For this review, take the finished solid that the model builds, in its own axes (mm). A direction names the side the tool comes from. Round coordinates to 2 decimals unless told otherwise and drop trailing zeros. Order: outer loops, then holes, each group sorted by start corner. A loop starts at its lowest first (then second) coordinate and runs counter-clockwise, first axis right, second up. Notation, with made-up numbers: M 65,-29 L 119,-29 A10 cw 119,-14 Z; hole C -26.5,87.25 d1. An arc over 180 degrees is marked long. Write item = value, one per line. Start each with the question number.
from build123d import *

# Parameters (mm, degrees)
SKETCH_1_R      = 50.5
SKETCH_1_R_2    = 2.6
SKETCH_1_R_3    = 35
EXTRUDE_1_DEPTH = 2
SKETCH_3_R      = 2.55
SKETCH_3_R_2    = 12
EXTRUDE_4_DEPTH = 2
FILLET_2_R      = 3


with BuildPart() as part:
    # 草图1 → 凸台-拉伸1 (new body)
    with BuildSketch(Plane.XY):
        Circle(SKETCH_1_R)
        with Locations((0, 40)):
            Circle(SKETCH_1_R_2, mode=Mode.SUBTRACT)
        Circle(SKETCH_1_R_3, mode=Mode.SUBTRACT)
        with Locations((28.284271247, 28.284271247)):
            Circle(SKETCH_1_R_2, mode=Mode.SUBTRACT)
        with Locations((40, 0)):
            Circle(SKETCH_1_R_2, mode=Mode.SUBTRACT)
        with Locations((28.284271247, -28.284271247)):
            Circle(SKETCH_1_R_2, mode=Mode.SUBTRACT)
        with Locations((0, -40)):
            Circle(SKETCH_1_R_2, mode=Mode.SUBTRACT)
        with Locations((-28.284271247, -28.284271247)):
            Circle(SKETCH_1_R_2, mode=Mode.SUBTRACT)
        with Locations((-40, 0)):
            Circle(SKETCH_1_R_2, mode=Mode.SUBTRACT)
        with Locations((-28.284271247, 28.284271247)):
            Circle(SKETCH_1_R_2, mode=Mode.SUBTRACT)
    extrude(amount=EXTRUDE_1_DEPTH)

    # 草图3 → 凸台-拉伸4 (add)
    with BuildSketch(Plane(origin=(0, 0, 0), x_dir=(-1, 0, 0), z_dir=(0, 0, -1))):
        with BuildLine():
            Line((-5, 34.641016151), (-5, 21.424285286))
            ThreePointArc((-5, 21.424285286), (-19.052558883, 11), (-21.053975315, -6.382015624))
            Line((-21.053975315, -6.382015624), (-32.5, -12.990381057))
            ThreePointArc((-32.5, -12.990381057), (-30.310889132, -17.5), (-27.5, -21.650635095))
            Line((-27.5, -21.650635095), (-16.053975315, -15.042269662))
            ThreePointArc((-16.053975315, -15.042269662), (0, -22), (16.053975315, -15.042269662))
            Line((16.053975315, -15.042269662), (27.5, -21.650635095))
            ThreePointArc((27.5, -21.650635095), (30.310889132, -17.5), (32.5, -12.990381057))
            Line((32.5, -12.990381057), (21.053975315, -6.382015624))
            ThreePointArc((21.053975315, -6.382015624), (19.052558883, 11), (5, 21.424285286))
            Line((5, 21.424285286), (5, 34.641016151))
            ThreePointArc((5, 34.641016151), (0, 35), (-5, 34.641016151))
        make_face()
        with Locations((0, 17.5)):
            Circle(SKETCH_3_R, mode=Mode.SUBTRACT)
        with Locations((0, -17.5)):
            Circle(SKETCH_3_R, mode=Mode.SUBTRACT)
        with Locations((-15.155444566, -8.75)):
            Circle(SKETCH_3_R, mode=Mode.SUBTRACT)
        with Locations((15.155444566, -8.75)):
            Circle(SKETCH_3_R, mode=Mode.SUBTRACT)
        with Locations((-15.155444566, 8.75)):
            Circle(SKETCH_3_R, mode=Mode.SUBTRACT)
        Circle(SKETCH_3_R_2, mode=Mode.SUBTRACT)
        with Locations((15.155444566, 8.75)):
            Circle(SKETCH_3_R, mode=Mode.SUBTRACT)
    extrude(amount=-EXTRUDE_4_DEPTH)

    # 圆角2
    fillet_2_edges = [part.edges().sort_by_distance(p)[0] for p in [
        (5, 21.424285286, 1),
        (5, 34.641016151, 1),
        (-5, 34.641016151, 1),
        (-5, 21.424285286, 1),
        (-21.053975315, -6.382015624, 1),
        (-32.5, -12.990381057, 1),
        (-27.5, -21.650635095, 1),
        (-16.053975315, -15.042269662, 1),
        (16.053975315, -15.042269662, 1),
        (27.5, -21.650635095, 1),
        (32.5, -12.990381057, 1),
        (21.053975315, -6.382015624, 1),
    ]]
    fillet(fillet_2_edges, radius=FILLET_2_R)


solid = part.part
(1) For line 1 along Y through (x, z) = (-25, 0.5); line 2 along X through (y, z) = (15.5, 1.4); line 3 along Y through (x, z) = (27, 0.2), list the stretches that pass through material, from the lowest coordinate up.
(2) We need section B-B, the plane x = 0. Write out the cut boundary in (y, z), then the cut area to 3 significant figures.
(3) Insertion check: pin 1 (4.5 mm diameter, centred on x = 28.28, y = 28.28, fed in from -Z); pin 2 (1 mm diameter, centred on y = 27, z = 1.5, fed in from -X). Each pin has a flat end and moves straight along its axis. Give the tip position at first contact, or say it passes through.
(4) For faces 1 (the flat face through (11, -11, 2)), 2 (the flat face through (21.217, -18.023, 0.986)), list the 3-axis set-ups (+Z, -Z, +X, -X, +Y, -Y) from which the entire face can be reached by the end or side of a thin tool; tool diameter is ignored.
(5) We need section A-A, the plane y = 0. Write out the cut boundary in (x, z).
(6) We need section D-D, the plane y = 17.5. Write out the cut boundary in (x, z).
(7) Draft analysis for pull direction X (two halves, no side actions). For faces 3 (the flat face through (11, -11, 0)), 4 (the flat face through (-26.217, -9.363, 0.986)), 5 (the cylindrical face through (29.68, -26.09, 0.99)), 6 (the cylindrical face through (-10.95, -49.3, 0.99)), state which applies: released by +X, released by -X, zero draft, split by the parting line, or undercut.
(8) We need section C-C, the plane y = 40. Write out the cut boundary in (x, z), then the cut area to 3 significant figures.
Values:
q1.line_1 = -43.88 to -24.49, -20.35 to -8.66, 24.49 to 43.88
q1.line_2 = -48.06 to -31.38, -15.61 to -1.58, 1.58 to 15.61, 31.38 to 48.06
q1.line_3 = -42.68 to -30.54, -26.02 to -9.81, 22.27 to 26.02, 30.54 to 42.68
q2.outline = M -50.5,0 L -42.6,0 L -42.6,2 L -50.5,2 Z; M -37.4,0 L -35,0 L -35,2 L -37.4,2 Z; M -22,0 L -20.05,0 L -20.05,2 L -22,2 Z; M -14.95,0 L -12,0 L -12,2 L -14.95,2 Z; M 12,0 L 14.95,0 L 14.95,2 L 12,2 Z; M 20.05,0 L 37.4,0 L 37.4,2 L 20.05,2 Z; M 42.6,0 L 50.5,0 L 50.5,2 L 42.6,2 Z
q2.area = 86.8 mm²
q3.pin_1 = through
q3.pin_2 = -42.99
q4.face_1 = +Z, +X, -X, +Y, -Y
q4.face_2 = +Z, -Z
q5.outline = M -50.5,0 L -42.6,0 L -42.6,2 L -50.5,2 Z; M -37.4,0 L -35,0 L -35,2 L -37.4,2 Z; M -22,0 L -12,0 L -12,2 L -22,2 Z; M 12,0 L 22,0 L 22,2 L 12,2 Z; M 35,0 L 37.4,0 L 37.4,2 L 35,2 Z; M 42.6,0 L 50.5,0 L 50.5,2 L 42.6,2 Z
q6.outline = M -47.37,0 L -30.31,0 L -30.31,2 L -47.37,2 Z; M -13.33,0 L -2.55,0 L -2.55,2 L -13.33,2 Z; M 2.55,0 L 13.33,0 L 13.33,2 L 2.55,2 Z; M 30.31,0 L 47.37,0 L 47.37,2 L 30.31,2 Z
q7.face_3 = zero draft
q7.face_4 = undercut
q7.face_5 = undercut
q7.face_6 = split by the parting line
q8.outline = M -30.83,0 L -2.6,0 L -2.6,2 L -30.83,2 Z; M 2.6,0 L 30.83,0 L 30.83,2 L 2.6,2 Z
q8.area = 113 mm²
